```python
from build123d import *

# Parameters (mm, degrees)
F1_DEPTH = 24.13
F2_R     = 4.7625
F3_R     = 4.7625
F4_DEPTH = 0.508
F5_W     = 13.716
F5_H     = 6.35
F5_W_2   = 8.128
F5_H_2   = 2.794
F6_DEPTH = 6.35


with BuildPart() as f1:
    # F0 (on Top) → F1 (new body)
    with BuildSketch(Plane.XY):
        with BuildLine():
            ThreePointArc((0, 9.525), (2.789808, 2.789808), (9.525, 0))
            Line((9.525, 0), (93.98, 0))
            ThreePointArc((93.98, 0), (100.715192, 2.789808), (103.505, 9.525))
            Line((103.505, 9.525), (103.505, 63.5))
            ThreePointArc((103.505, 63.5), (100.715192, 70.235192), (93.98, 73.025))
            Line((93.98, 73.025), (9.525, 73.025))
            ThreePointArc((9.525, 73.025), (2.789808, 70.235192), (0, 63.5))
            Line((0, 63.5), (0, 9.525))
        make_face()
    extrude(amount=F1_DEPTH)

    # F2
    f2_edges = [f1.edges().sort_by_distance(p)[0] for p in [
        (0, 36.5125, 24.13),
        (2.789808, 2.789808, 24.13),
        (51.7525, 0, 24.13),
        (100.715192, 2.789808, 24.13),
        (103.505, 36.5125, 24.13),
        (100.715192, 70.235192, 24.13),
        (51.7525, 73.025, 24.13),
        (2.789808, 70.235192, 24.13),
        (0, 36.5125, 0),
        (2.789808, 2.789808, 0),
        (51.7525, 0, 0),
        (100.715192, 2.789808, 0),
        (103.505, 36.5125, 0),
        (100.715192, 70.235192, 0),
        (51.7525, 73.025, 0),
        (2.789808, 70.235192, 0),
    ]]
    fillet(f2_edges, radius=F2_R)

    # F3 (on face) → F4 (cut)
    with BuildSketch(Plane.XY.offset(24.13)):
        with Locations((12.7, 36.5125)):
            Circle(F3_R)
    extrude(amount=-F4_DEPTH, mode=Mode.SUBTRACT)

    # F5 (on face) → F6 (cut)
    with BuildSketch(Plane(origin=(0, 0, 0), x_dir=(0, -1, 0), z_dir=(-1, 0, 0))):
        with Locations((-51.3715, 12.065)):
            Rectangle(F5_W, F5_H)
        with Locations((-36.5125, 15.113)):
            Rectangle(F5_W_2, F5_H_2)
        with Locations((-21.6535, 12.065)):
            Rectangle(F5_W, F5_H)
    extrude(amount=-F6_DEPTH, mode=Mode.SUBTRACT)


solid = f1.part
```
Can you work these out from the model? Positions are in its coordinate system, mm. A direction names the side the tool comes from. Coordinates: 2 decimals unless noted, no trailing zeros.
1. I need wall thicknesses on line 1 (X direction, y = 25, z = 11) (3 decimals); line 2 (X direction, y = 25, z = 19.5); line 3 (Y direction, x = 77.5, z = 4.5). Which ranges of each line are inside material? Lowest first, please.
2. I'm going to push flat-ended pins straight in: pin 1 (5 mm diameter, centred on x = 2, y = 38.5, fed in from -Z); pin 2 (2 mm diameter, centred on y = 43.5, z = 21, fed in from -X); pin 3 (1.9 mm diameter, centred on y = 24.5, z = 13, fed in from -X). Where does each tip first touch, or does it pass through?
3. Thinking about a two-plate mould opening in Z: for faces 4 (the face through (6.35, 51, 12)), 5 (the face through (1.36, 36.13, 22.7)), 6 (the face through (3, 58.229, 12)), 7 (the face through (52, 73.025, 12)), which applies, +Z half, -Z half, draft (parallel to the pull), parting line (faces both ways), or undercut?
4. For faces 1 (the face through (6.35, 37, 15)), 2 (the face through (51, 0, 12)), 3 (the face through (13, 37, 23.622)), which set-ups out of +Z, -Z, +X, -X, +Y, -Y let a thin tool reach every point of the face, with its end or its side?
Entries:
1. line 1: x = 6.35 to 103.505
1. line 2: x = 0 to 103.5
1. line 3: y = 0.01 to 73.02
2. pin 1: stops at z = 0.01
2. pin 2: stops at x = 0.04
2. pin 3: stops at x = 6.35
3. face 4: undercut
3. face 5: +Z half
3. face 6: undercut
3. face 7: draft
4. face 1: -X
4. face 2: +Z, -Z, +X, -X, -Y
4. face 3: +Z
